The model under review builds one solid part; all positions refer to its coordinate system, in mm. Coordinates: 2 decimals unless noted, no trailing zeros. Put each result on its own line as item: value. Start each with the question number.
Item 1: To check wall thickness, follow L1, parallel to Y at x = -13, z = 572.5; L2, parallel to X at y = -16, z = 211. State the ranges of each line that lie inside material, in increasing order. Write a range as [from, to].
Item 2: Consider section A-A on z = 292. State how many separate pieces and enclosed holes the cut face has, then the cut area to 3 significant figures.
Item 3: For pin 1 (3 mm diameter, centred on y = -1, z = 282, fed in from +X); pin 2 (3 mm diameter, centred on x = -0.5, z = 559, fed in from +Y), all flat-tipped, find the tip position at first contact; note any pin that passes through.
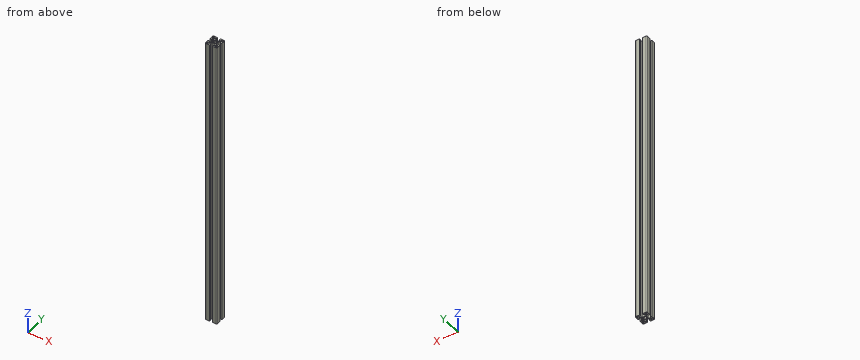
Autodesk Inventor part; units mm, degrees
ref_plane "YZ Plane" through (0, 0, 0) normal (1, 0, 0) x (0, 1, 0)
ref_plane "XZ Plane" through (0, 0, 0) normal (0, 1, 0) x (-1, 0, 0)
ref_plane "XY Plane" through (0, 0, 0) normal (0, 0, 1) x (1, 0, 0)
sketch "T-Slot 4040 Base" plane through (0, 0, 0) normal (0, 0, 1) x (1, 0, 0)
  line L0 (-28, 0) -> (28, 0) construction
  line L1 (0, -28) -> (0, 28) construction
  circle A0 centre (0, 0) radius 5.1
  line L2 (-7.5, -7.5) -> (7.5, -7.5)
  line L3 (7.5, -7.5) -> (7.5, 7.5)
  line L4 (7.5, 7.5) -> (-7.5, 7.5)
  line L5 (-7.5, 7.5) -> (-7.5, -7.5)
  line L6 (-7.5, -7.5) -> (7.5, 7.5) construction
  line L7 (7.5, -7.5) -> (-7.5, 7.5) construction
  line L8 (-20, 20) -> (20, 20)
  line L9 (20, 20) -> (20, -20)
  line L10 (20, -20) -> (-20, -20)
  line L11 (-20, -20) -> (-20, 20)
  line L12 (-20, 20) -> (20, -20) construction
  line L13 (20, 20) -> (-20, -20) construction
  line L14 (20, 5) -> (14.5, 5)
  line L15 (14.5, 5) -> (14.5, 10)
  line L16 (14.5, 10) -> (12.4749, 10)
  line L17 (12.4749, 10) -> (7.5, 5.0251)
  line L18 (5, 20) -> (5, 14.5)
  line L19 (5, 14.5) -> (10, 14.5)
  line L20 (10, 14.5) -> (10, 12.4749)
  line L21 (10, 12.4749) -> (5.0251, 7.5)
  line L22 (18.5, 18.5) -> (11.5, 18.5)
  line L23 (11.5, 18.5) -> (11.5, 11.5)
  line L24 (11.5, 11.5) -> (18.5, 11.5)
  line L25 (18.5, 11.5) -> (18.5, 18.5)
  line L26 (18.5, 18.5) -> (11.5, 11.5) construction
  line L27 (11.5, 18.5) -> (18.5, 11.5) construction
  line L28 (3.0732, 1.3088) -> (4.38, 2.6125) construction
  line L29 (5.905, 4.1338) -> (4.1393, 5.9037)
  line L30 (4.1393, 5.9037) -> (2.6122, 4.3802)
  line L31 (1.3075, 3.0787) -> (3.0732, 1.3088) construction
  line L32 (3.0732, 1.3088) -> (4.1393, 5.9037) construction
  line L33 (5.905, 4.1338) -> (1.3075, 3.0787) construction
  line L34 (4.38, 2.6125) -> (5.905, 4.1338)
  line L35 (2.6122, 4.3802) -> (1.3075, 3.0787) construction
  line L36 (-20, 5) -> (-14.5, 5)
  line L37 (-14.5, 5) -> (-14.5, 10)
  line L38 (-14.5, 10) -> (-12.4749, 10)
  line L39 (-12.4749, 10) -> (-7.5, 5.0251)
  line L40 (-5, 20) -> (-5, 14.5)
  line L41 (-5, 14.5) -> (-10, 14.5)
  line L42 (-10, 14.5) -> (-10, 12.4749)
  line L43 (-10, 12.4749) -> (-5.0251, 7.5)
  line L44 (-18.5, 18.5) -> (-11.5, 18.5)
  line L45 (-11.5, 18.5) -> (-11.5, 11.5)
  line L46 (-11.5, 11.5) -> (-18.5, 11.5)
  line L47 (-18.5, 11.5) -> (-18.5, 18.5)
  line L48 (-5.905, 4.1338) -> (-4.1393, 5.9037)
  line L49 (-4.1393, 5.9037) -> (-2.6122, 4.3802)
  line L50 (-4.38, 2.6125) -> (-5.905, 4.1338)
  line L51 (7.5, -7.5) -> (-7.5, -7.5)
  line L52 (20, -5) -> (14.5, -5)
  line L53 (14.5, -5) -> (14.5, -10)
  line L54 (14.5, -10) -> (12.4749, -10)
  line L55 (12.4749, -10) -> (7.5, -5.0251)
  line L56 (5, -20) -> (5, -14.5)
  line L57 (5, -14.5) -> (10, -14.5)
  line L58 (10, -14.5) -> (10, -12.4749)
  line L59 (10, -12.4749) -> (5.0251, -7.5)
  line L60 (18.5, -18.5) -> (11.5, -18.5)
  line L61 (11.5, -18.5) -> (11.5, -11.5)
  line L62 (11.5, -11.5) -> (18.5, -11.5)
  line L63 (18.5, -11.5) -> (18.5, -18.5)
  line L64 (18.5, -18.5) -> (11.5, -11.5) construction
  line L65 (11.5, -18.5) -> (18.5, -11.5) construction
  line L66 (3.0732, -1.3088) -> (4.38, -2.6125) construction
  line L67 (5.905, -4.1338) -> (4.1393, -5.9037)
  line L68 (4.1393, -5.9037) -> (2.6122, -4.3802)
  line L69 (1.3075, -3.0787) -> (3.0732, -1.3088) construction
  line L70 (3.0732, -1.3088) -> (4.1393, -5.9037) construction
  line L71 (5.905, -4.1338) -> (1.3075, -3.0787) construction
  line L72 (4.38, -2.6125) -> (5.905, -4.1338)
  line L73 (2.6122, -4.3802) -> (1.3075, -3.0787) construction
  line L74 (-4.38, -2.6125) -> (-5.905, -4.1338)
  line L75 (-4.1393, -5.9037) -> (-2.6122, -4.3802)
  line L76 (-5.905, -4.1338) -> (-4.1393, -5.9037)
  line L77 (-12.4749, -10) -> (-7.5, -5.0251)
  line L78 (-10, -12.4749) -> (-5.0251, -7.5)
  line L79 (-10, -14.5) -> (-10, -12.4749)
  line L80 (-5, -14.5) -> (-10, -14.5)
  line L81 (-5, -20) -> (-5, -14.5)
  line L82 (-18.5, -18.5) -> (-11.5, -18.5)
  line L83 (-11.5, -18.5) -> (-11.5, -11.5)
  line L84 (-11.5, -11.5) -> (-18.5, -11.5)
  line L85 (-18.5, -11.5) -> (-18.5, -18.5)
  line L86 (-14.5, -10) -> (-12.4749, -10)
  line L87 (-14.5, -5) -> (-14.5, -10)
  line L88 (-20, -5) -> (-14.5, -5)
  point P0 (15, 15)
  point P1 (3.6062, 3.6062)
  point P2 (3.6062, 3.6062)
  point P3 (15, -15)
  point P4 (3.6062, -3.6062)
  point P5 (3.6062, -3.6062)
  dimension "d9" = 10.2
  dimension "d12" = 40
  dimension "d13" = 40
  dimension "d14" = 5.5
  dimension "d15" = 15
  dimension "d16" = 7
  dimension "d17" = 10
  dimension "d20" = 1.75
  dimension "d21" = 7
  dimension "d22" = 2
  dimension "d29" = 1.5
  dimension "d30" = 2.5
extrude "Extrusion1" add sketch "T-Slot 4040 Base" along normal blind 1000 contours L5 L4 L3 L2 | L2 L78 L79 L80 L81 L10 L11 L88 L87 L86 L77 L5 | L2 L3 L55 L54 L53 L52 L9 L10 L56 L57 L58 L59 | L39 L38 L37 L36 L11 L8 L40 L41 L42 L43 L4 L5 | L3 L4 L21 L20 L19 L18 L8 L9 L14 L15 L16 L17
fillet "Rundung1" radius 1 16 edges at (11.5, 18.5, 500) (18.5, 18.5, 500) (18.5, 11.5, 500) (11.5, 11.5, 500) (-11.5, 18.5, 500) (-18.5, 18.5, 500) (-18.5, 11.5, 500) (-11.5, 11.5, 500) (-18.5, -11.5, 500) (-11.5, -11.5, 500) (-11.5, -18.5, 500) (-18.5, -18.5, 500) (11.5, -18.5, 500) (11.5, -11.5, 500) (18.5, -11.5, 500) (18.5, -18.5, 500)
fillet "Rundung2" radius 3 4 edges at (20, 20, 500) (20, -20, 500) (-20, -20, 500) (-20, 20, 500)
properties part number "T-SLOT 4040 B-Type 1000mm"
Report:
1. L1: [-20, -18.5], [-11.5, -10], [10, 11.5], [18.5, 20]
1. L2: [-20, -18.5], [-11.5, -5], [5, 11.5], [18.5, 20]
2. separate pieces: 1
2. enclosed holes: 5
2. area: 616 mm²
3. pin 1: x = 7.5
3. pin 2: y = 7.5
